CAD build for the part. Positions are in the model's coordinates, mm. A direction names the side the tool comes from. Coordinates: 2 decimals unless noted, no trailing zeros. Order: outer loops, then holes, each group sorted by start corner. A loop starts at its lowest first (then second) coordinate and runs counter-clockwise, first axis right, second up. Notation, with made-up numbers: M 82.25,40.25 L 90.25,40.25 A17 ccw 90.25,70.25 Z; hole C 4,63 d9. An arc over 180 degrees is marked long. Write item = value, one per line.
from build123d import *

# Parameters (mm, degrees)
F0_R     = 40
F1_DEPTH = 200
F2_R     = 5
F3_R     = 36.5
F4_DEPTH = 192


with BuildPart() as f1:
    # F0 (on Top) → F1 (new body)
    with BuildSketch(Plane.XY):
        Circle(F0_R)
    extrude(amount=F1_DEPTH)

    # F2
    f2_edges = [f1.edges().sort_by_distance(p)[0] for p in [
        (-40, 0, 0),
    ]]
    fillet(f2_edges, radius=F2_R)

    # F3 (on face) → F4 (cut)
    with BuildSketch(Plane.XY.offset(200)):
        Circle(F3_R)
    extrude(amount=-F4_DEPTH, mode=Mode.SUBTRACT)


solid = f1.part
(1) Wall check: line 1 (Y direction, x = 0, z = 103.5); line 2 (Z direction, x = 23, y = -2); line 3 (X direction, y = 30, z = 56). Give the ranges that are in metal, low to high. Write a range as from..to.
Evaluation:
line_1 = -40..-36.5, 36.5..40
line_2 = 0..8
line_3 = -26.46..-20.79, 20.79..26.46
(2) Pin check, flat tips, straight feed: pin 1 Ø3 at (y, z) = (23.5, 30.5) entering from +X; pin 2 Ø5 at (y, z) = (29, 77.5) entering from +X; pin 3 Ø5 at (x, y) = (-18, 22.5) entering from -Z; pin 4 Ø8 at (x, y) = (18, 2.5) entering from +Z. Stop position of each tip, or through.
Evaluation:
pin_1 = 33.41
pin_2 = 29.96
pin_3 = 0
pin_4 = 8
(3) Slice it at A-A, the plane x = 0. Write the cut outline in (y, z).
Evaluation:
outline = M -40,5 A5 ccw -35,0 L 35,0 A5 ccw 40,5 L 40,200 L 36.5,200 L 36.5,8 L -36.5,8 L -36.5,200 L -40,200 Z
(4) Pull direction Y, two halves, no side cores. Call faces 1 (the face through (-8.67, -39.05, 101.14)), 2 (the face through (-7.912, -35.632, 105.344)), 3 (the face through (0, 0, 0)): +Y half, -Y half, draft (parallel to the pull), parting line (faces both ways), or undercut.
Evaluation:
face_1 = parting line
face_2 = undercut
face_3 = draft
(5) Tool access for faces 4 (the face through (32, -18, 200)), 5 (the face through (-1, 1, 8)): list every direction of +Z, -Z, +X, -X, +Y, -Y with a clear straight run to the whole face (end or side of a thin tool).
Evaluation:
face_4 = +Z, +X, -X, +Y, -Y
face_5 = +Z
(6) Slice it at B-B, the plane z = 180. Write the cut outline in (x, y).
Evaluation:
outline = C 0,0 d80; hole C 0,0 d73
